```python
from build123d import *

# Parameters (mm, degrees)
EXTRUDE1_DEPTH     = 25
SKETCH2_R          = 3.15
CUT_EXTRUDE1_DEPTH = 25
SKETCH3_R          = 3.15
CUT_EXTRUDE2_DEPTH = 25


with BuildPart() as part:
    # Sketch1 → Extrude1 (new body)
    with BuildSketch(Plane.XY):
        with BuildLine():
            Line((22.39626556, -5.458921162), (22.39626556, -30.458921162))
            Line((22.39626556, -30.458921162), (-2.60373444, -30.458921162))
            ThreePointArc((-2.60373444, -30.458921162), (-1.725054783, -28.337600818), (0.39626556, -27.458921162))
            Line((0.39626556, -27.458921162), (16.39626556, -27.458921162))
            ThreePointArc((16.39626556, -27.458921162), (18.517585904, -26.580241505), (19.39626556, -24.458921162))
            Line((19.39626556, -24.458921162), (19.39626556, -8.458921162))
            ThreePointArc((19.39626556, -8.458921162), (20.274945217, -6.337600818), (22.39626556, -5.458921162))
        make_face()
    extrude(amount=EXTRUDE1_DEPTH)

    # Sketch2 → Cut-Extrude1 (cut)
    with BuildSketch(Plane(origin=(22.39626556, 0, 0), x_dir=(0, 0, -1), z_dir=(1, 0, 0))):
        with Locations(Location((-12.5, -17.958921162, 0), (0, 0, 90))):
            Circle(SKETCH2_R)
    extrude(amount=-CUT_EXTRUDE1_DEPTH, mode=Mode.SUBTRACT)

    # Sketch3 → Cut-Extrude2 (cut)
    with BuildSketch(Plane.XZ.offset(30.458921162)):
        with Locations(Location((9.89626556, 12.5, 0), (0, 0, 270))):
            Circle(SKETCH3_R)
    extrude(amount=-CUT_EXTRUDE2_DEPTH, mode=Mode.SUBTRACT)


solid = part.part
```
Design review of the part built by this model. Coordinates are the model's own, in mm. A direction names the side the tool comes from. Coordinates: 2 decimals unless noted, no trailing zeros. Order: outer loops, then holes, each group sorted by start corner. A loop starts at its lowest first (then second) coordinate and runs counter-clockwise, first axis right, second up. Notation, with made-up numbers: M 20.5,48.5 L 37.5,48.5 A22 ccw 37.5,55.5 Z; hole C 63,68.25 d10. An arc over 180 degrees is marked long. Answer as a JSON object with one key per item and string values. Group by question number.
1) Add section A-A, the plane z = 12.5. Write out the cut boundary in (x, y).
2) Add section B-B, the plane z = 6. Write out the cut boundary in (x, y), then the cut area to 3 significant figures.
3) Wall thickness on L1, parallel to Z at x = 9.75, y = -28.5; L2, parallel to X at y = -28.05, z = 12.5; L3, parallel to X at y = -11, z = 11: over which ranges is each line inside the solid? List them lowest first.
4) For pin 1 (5 mm diameter, centred on x = 8, z = 14, fed in from +Y); pin 2 (13 mm diameter, centred on y = -16.5, z = 10, fed in from -X), all flat-tipped, find the tip position at first contact; note any pin that passes through.
5) Mouldability with a two-part tool opening along Z and no side actions: class faces 3 (the cylindrical face through (12.025, -28.98, 14.822)), 4 (the flat face through (16, -28, 0)), 5 (the flat face through (16, -28, 25)), 6 (the cylindrical face through (20.917, -14.954, 13.446)) as pulls with the +Z half, pulls with the -Z half, needs draft (parallel to the pull), parting line crosses it, or undercut.
6) Tool access review of faces 1 (the flat face through (22.396, -15, 10)), 2 (the flat face through (19.396, -15, 10)): name each direction out of +Z, -Z, +X, -X, +Y, -Y from which nothing blocks a thin tool from reaching the whole face with its end or side.
7) Add section C-C, the plane x = 7.75. Write out the cut boundary in (y, z), then the cut area to 3 significant figures.
8) Add section D-D, the plane y = -28.5. Write out the cut boundary in (x, z).
Computed values:
{
 "1": {"outline": "M -2.6,-30.46 L 6.75,-30.46 L 6.75,-27.46 L 0.4,-27.46 A3 ccw Z; M 13.05,-30.46 L 22.4,-30.46 L 22.4,-21.11 L 19.4,-21.11 L 19.4,-24.46 A3 cw 16.4,-27.46 L 13.05,-27.46 Z; M 19.4,-14.81 L 22.4,-14.81 L 22.4,-5.46 A3 ccw 19.4,-8.46 Z"},
 "2": {"outline": "M -2.6,-30.46 L 22.4,-30.46 L 22.4,-5.46 A3 ccw 19.4,-8.46 L 19.4,-24.46 A3 cw 16.4,-27.46 L 0.4,-27.46 A3 ccw Z", "area": "139 mm^2"},
 "3": {"L1": "z = 0 to 9.35, 15.65 to 25", "L2": "x = -1.39 to 6.75, 13.05 to 22.4", "L3": "x = 19.4 to 22.4"},
 "4": {"pin 1": "stops at y = -27.46", "pin 2": "stops at x = 19.4"},
 "5": {"face 3": "undercut", "face 4": "pulls with the -Z half", "face 5": "pulls with the +Z half", "face 6": "undercut"},
 "6": {"face 1": "+Z, -Z, +X, +Y, -Y", "face 2": "+Z, -Z, -X, +Y"},
 "7": {"outline": "M -30.46,0 L -27.46,0 L -27.46,10.19 L -30.46,10.19 Z; M -30.46,14.81 L -27.46,14.81 L -27.46,25 L -30.46,25 Z", "area": "61.2 mm^2"},
 "8": {"outline": "M -1.88,0 L 22.4,0 L 22.4,25 L -1.88,25 Z; hole C 9.9,12.5 d6.3"}
}
